Autodesk Inventor part; units mm, degrees
ref_plane "YZ Plane" through (0, 0, 0) normal (1, 0, 0) x (0, 1, 0)
ref_plane "XZ Plane" through (0, 0, 0) normal (0, 1, 0) x (-1, 0, 0)
ref_plane "XY Plane" through (0, 0, 0) normal (0, 0, 1) x (1, 0, 0)
sketch "Sketch1" plane through (0, 0, 0) normal (1, 0, 0) x (0, 1, 0)
  line L0 (-8.5, 12.5) -> (8.5, 12.5)
  line L1 (8.5, 12.5) -> (8.5, -12.5)
  line L2 (8.5, -12.5) -> (-8.5, -12.5)
  line L3 (-8.5, -12.5) -> (-8.5, 12.5)
  line L4 (-8.5, 12.5) -> (8.5, -12.5) construction
  line L5 (8.5, 12.5) -> (-8.5, -12.5) construction
  line L6 (8.5, -12.5) -> (33.5, -12.5)
  line L7 (8.5, -12.5) -> (33.5, -12.5) construction
  line L8 (33.5, -12.5) -> (33.5, -4.25)
  line L9 (33.5, -4.25) -> (8.5, -4.25)
  line L10 (33.5, -4.25) -> (58.5, -4.25) construction
  point P0 (0, 0)
  dimension "d0" = 17
  dimension "d1" = 25
  dimension "d2" = 25
  dimension "d3" = 0
  dimension "d4" = 8.25
  dimension "d5" = 90
  dimension "d6" = 180
extrude "Extrusion1" add sketch "Sketch1" along normal blind 20
sketch "Sketch2" plane through (0, 8.5, -4.25) normal (0, 0, 1) x (1, 0, 0)
  circle A0 centre (10, 10.5) radius 3.81
  line L0 (0, 25) -> (20, 25)
  line L1 (0, -8.5) -> (20, -8.5) construction
  line L2 (20, -17) -> (20, 25)
  dimension "d9" = 7.62
  dimension "d32" = 19
extrude "Extrusion2" cut sketch "Sketch2" against normal through all
sketch "Sketch3" plane through (0, 8.5, -4.25) normal (0, 0, 1) x (1, 0, 0)
  circle A0 centre (10, 10.5) radius 3.81
  circle A1 centre (10, 10.5) radius 4.815
  point P0 (0, -8.5)
  dimension "d13" = 9.63
extrude "Extrusion3" cut sketch "Sketch3" against normal blind 3.2
sketch "Sketch4" plane through (0, 8.5, -4.25) normal (0, 0, 1) x (1, 0, 0)
  circle A0 centre (10, 10.5) radius 3.81
  circle A1 centre (10, 10.5) radius 5.39
  point P0 (0, -8.5)
  dimension "d16" = 10.78
extrude "Extrusion4" cut sketch "Sketch4" against normal blind 0.92
sketch "Sketch6" plane through (0, -8.5, -12.5) normal (0, -1, 0) x (1, 0, 0)
  circle A0 centre (10, 12) radius 6.2485
  line L0 (0, 0) -> (20, 0)
  line L1 (0, 25) -> (0, 0)
  point P0 (0, 12.5)
  dimension "d22" = 12.497
  dimension "d25" = 12
  dimension "d26" = 10
extrude "Extrusion6" [suppressed]
sketch "Sketch9" plane through (0, -8.5, -12.5) normal (0, 0, -1) x (-1, 0, 0)
  line L0 (-5, 20) -> (-15, 20)
  line L1 (-15, 20) -> (-15, 10)
  line L2 (-15, 10) -> (-5, 10)
  line L3 (-5, 10) -> (-5, 20)
  line L4 (0, 0) -> (0, 42)
  line L5 (0, 0) -> (-20, 0)
  point P0 (0, 8.5)
  dimension "d38" = 10
  dimension "d39" = 10
  dimension "d40" = 5
  dimension "d41" = 10
extrude "Extrusion8" add sketch "Sketch9" along normal blind 6.35
sketch "Sketch12" plane through (20, 0, 0) normal (1, 0, 0) x (0, 0, -1)
  line L0 (12.5, -8.5) -> (12.5, 33.5)
  line L1 (12.5, 33.5) -> (4.25, 33.5)
  line L2 (4.25, 33.5) -> (4.25, 8.5)
  line L3 (4.25, 8.5) -> (-12.5, 8.5)
  line L4 (-12.5, 8.5) -> (-12.5, -8.5)
  line L5 (-12.5, -8.5) -> (12.5, -8.5)
  line L6 (-12.5, -8.5) -> (12.5, -8.5)
  line L7 (12.5, -8.5) -> (-12.5, -8.5)
  line L8 (-12.5, -8.5) -> (-12.5, 33.5)
  line L9 (-12.5, 33.5) -> (12.5, 33.5)
  line L10 (12.5, 33.5) -> (12.5, -8.5)
  line L11 (12.5, 33.5) -> (4.25, 33.5)
  line L12 (-12.5, 8.5) -> (-12.5, -8.5)
  point P0 (0, 0)
extrude "Extrusion10" add sketch "Sketch12" along normal blind 5
sketch "Sketch14" plane through (0, 0, 0) normal (-1, 0, 0) x (0, 0, 1)
  circle A0 centre (3.3578, 0) radius 4.1
  line L0 (-12.5, -8.5) -> (-12.5, 33.5)
  line L1 (12.5, -8.5) -> (-12.5, -8.5)
  line L2 (12.5, 8.5) -> (12.5, -8.5)
  line L3 (-4.25, 8.5) -> (12.5, 8.5)
  line L4 (-4.25, 33.5) -> (-4.25, 8.5)
  line L5 (-12.5, 33.5) -> (-4.25, 33.5)
  point P0 (0, 0)
  dimension "d52" = 8.5
  dimension "d53" = 8.2
extrude "Extrusion11" cut sketch "Sketch14" against normal blind 10.2 contours A0
sketch "Sketch15" plane through (25, 0, 0) normal (1, 0, 0) x (0, 0, -1)
  line L0 (12.5, -8.5) -> (12.5, 33.5)
  line L1 (12.5, 33.5) -> (-12.5, 33.5)
  line L2 (-12.5, 33.5) -> (-12.5, -8.5)
  line L3 (-12.5, -8.5) -> (12.5, -8.5)
  circle A0 centre (-3.3578, 0) radius 4.1
  circle A1 centre (-3.3578, 0) radius 4.1
  line L4 (-5.5, -0.5) -> (4.5, -0.5)
  line L5 (4.5, -0.5) -> (4.5, 9.5)
  line L6 (4.5, 9.5) -> (-5.5, 9.5)
  line L7 (-5.5, 9.5) -> (-5.5, -0.5)
  line L8 (-5.5, -0.5) -> (4.5, 9.5) construction
  line L9 (4.5, -0.5) -> (-5.5, 9.5) construction
  point P0 (0, 0)
  point P1 (-0.5, 4.5)
  dimension "d56" = 10
  dimension "d57" = 10
  dimension "d58" = 8
  dimension "d59" = 8
extrude "Extrusion12" add sketch "Sketch15" along normal blind 6.35 contours A0 L4 L7 | A0 L7 L6 L5 L4 picked at (-1.3763, 0.1524)
fillet "Fillet3" radius 2 9 edges at (0, 21, -4.25) (0, 8.5, 4.125) (10, 8.5, 12.5) (0, 0, 12.5) (20, 21, 12.5) (20, 33.5, 4.125) (10, 33.5, -4.25) (12.5, -8.5, 12.5) (0, -8.5, 0)
sketch "Sketch10" plane through (0, 0, 0) normal (-1, 0, 0) x (0, 0, 1)
  line L0 (-12.5, -8.5) -> (-12.5, 33.5)
  line L1 (12.5, -8.5) -> (-12.5, -8.5)
  line L2 (12.5, 8.5) -> (12.5, -8.5)
  line L3 (-4.25, 8.5) -> (12.5, 8.5)
  line L4 (-4.25, 33.5) -> (-4.25, 8.5)
  line L5 (-12.5, 33.5) -> (-4.25, 33.5)
  line L6 (2.5, 6.5) -> (-7.5, 6.5)
  line L7 (-7.5, 6.5) -> (-7.5, -3.5)
  line L8 (-7.5, -3.5) -> (2.5, -3.5)
  line L9 (2.5, -3.5) -> (2.5, 6.5)
  point P0 (0, 0)
  dimension "d44" = 10
  dimension "d45" = 10
  dimension "d46" = 5
  dimension "d47" = 5
sketch "Sketch8" plane through (20, 0, 0) normal (1, 0, 0) x (0, 0, -1)
  circle A0 centre (-2, 0) radius 4.05
  line L0 (4.25, 13.61) -> (4.25, 24.39)
  line L1 (4.25, 10.5) -> (4.25, 31.5)
  line L2 (4.25, 31.5) -> (4.25, 10.5)
  line L3 (7.45, 22.81) -> (7.45, 15.19)
  line L4 (12.5, 22.81) -> (12.5, 15.19)
  line L5 (7.45, 22.81) -> (7.45, 15.19)
  point P0 (0, 0)
  dimension "d34" = 8.1
  dimension "d35" = 6.25
sketch "Sketch5" plane through (20, 0, 0) normal (1, 0, 0) x (0, 0, -1)
  circle A0 centre (0, 0) radius 4.05
  line L0 (27.5, -8.5) -> (27.5, 33.5)
  line L1 (27.5, 33.5) -> (19.5, 33.5)
  line L2 (19.5, 33.5) -> (19.5, 8.5)
  line L3 (19.5, 8.5) -> (-27.5, 8.5)
  line L4 (-27.5, 8.5) -> (-27.5, -8.5)
  line L5 (-27.5, -8.5) -> (27.5, -8.5)
  dimension "d19" = 8.1
  dimension "d33" = 27.5
properties part number "frame-holder-v3"
Part model, mm, in its own coordinate system. A direction names the side the tool comes from. Round coordinates to 2 decimals unless told otherwise and drop trailing zeros. Loops run counter-clockwise (first coordinate to the right, second up) from the corner with the lowest first, then second, coordinate; pieces in that order, holes last. Notation, with made-up numbers: (14, -20) - (65, -20) arc R7 ccw to (65, -15) - close; hole circle Ø6 at (48.25, 5). An arc over 180 degrees is marked (long way). Answer as a JSON object with one key per item and string values.
Item 1: Pin check, flat tips, straight feed: pin 1 (5 mm diameter, centred on x = 10.5, z = -16.5, fed in from -Y); pin 2 (7.5 mm diameter, centred on y = 24.5, z = 0, fed in from -X); pin 3 (16 mm diameter, centred on x = 14.5, z = 3, fed in from +Y); pin 4 (3 mm diameter, centred on y = 5.5, z = -17, fed in from -X). Stop position of each tip, or through.
Output:
{"pin 1": "y = 1.5", "pin 2": "x = 20", "pin 3": "y = 33.5", "pin 4": "x = 5"}
Item 2: Band-saw the part on D-D on y = 28. List the corners of the cut face in (x, z).
Output:
{"outline": "(0, -12.5) - (25, -12.5) - (25, 12.5) - (22, 12.5) arc R2 ccw to (20, 10.5) - (20, -4.25) - (2, -4.25) arc R2 ccw to (0, -6.25) - close"}
Item 3: Pull direction Z, two halves, no side cores. Call faces 1 (the face through (28, -0.5, 1)), 2 (the face through (20.6, 19.81, 11.93)), 3 (the face through (5.03, 0.18, -0.74)), 4 (the face through (10.2, 0, 3)): pulls with the +Z half, pulls with the -Z half, needs draft (parallel to the pull), parting line crosses it, or undercut.
Output:
{"face 1": "needs draft", "face 2": "pulls with the +Z half", "face 3": "undercut", "face 4": "undercut"}
Item 4: Band-saw the part on C-C on x = 16.5. List the corners of the cut face in (y, z), plus the area to 3 significant figures.
Output:
{"outline": "(-8.5, -12.5) - (33.5, -12.5) - (33.5, -6.25) arc R2 ccw to (31.5, -4.25) - (8.5, -4.25) - (8.5, 10.5) arc R2 ccw to (6.5, 12.5) - (-6.5, 12.5) arc R2 ccw to (-8.5, 10.5) - close", "area": "629 mm2"}
Item 5: Tool access for faces 5 (the face through (13.66, -7.9, 11.93)), 6 (the face through (20.57, 32.9, 2.99)), 7 (the face through (14, 20, -7.45)), 8 (the face through (10, 1.5, -16)), 9 (the face through (15, 7, -16)): list every direction of +Z, -Z, +X, -X, +Y, -Y with a clear straight run to the whole face (end or side of a thin tool).
Output:
{"face 5": "+Z, +X, -X, -Y", "face 6": "+Z, -X, +Y", "face 7": "+Z", "face 8": "-Z, +X, -X, -Y", "face 9": "-Z, +X, +Y, -Y"}
Item 6: Band-saw the part on A-A on y = 19. List the corners of the cut face in (x, z) (3 decimals), plus the area to 3 significant figures.
Output:
{"outline": "(0, -12.5) - (6.19, -12.5) - (6.19, -7.45) - (5.185, -7.45) - (5.185, -5.17) - (4.61, -5.17) - (4.61, -4.25) - (2, -4.25) arc R2 ccw to (0, -6.25) - close; (13.81, -12.5) - (25, -12.5) - (25, 12.5) - (22, 12.5) arc R2 ccw to (20, 10.5) - (20, -4.25) - (15.39, -4.25) - (15.39, -5.17) - (14.815, -5.17) - (14.815, -7.45) - (13.81, -7.45) - close", "area": "218 mm2"}
Item 7: Wall check: L1, parallel to Y at x = 10, z = -6.6 (3 decimals); L2, parallel to X at y = 22, z = 7.5; L3, parallel to Y at x = 10, z = -10. Give the ranges that are in metal, low to high.
Output:
{"L1": "-8.5 to 14.185, 23.815 to 33.5", "L2": "20 to 25", "L3": "-8.5 to 15.19, 22.81 to 33.5"}
Item 8: Band-saw the part on B-B on z = -2.5. List the corners of the cut face in (x, y).
Output:
{"outline": "(0, -6.5) arc R2 ccw to (2, -8.5) - (25, -8.5) - (25, -0.5) - (31.35, -0.5) - (31.35, 9.5) - (25, 9.5) - (25, 33.5) - (22, 33.5) arc R2 ccw to (20, 31.5) - (20, 8.5) - (2, 8.5) arc R2 ccw to (0, 6.5) - close"}
